```python
from build123d import *

# Parameters (mm, degrees)
F1_DEPTH       = 59.9186
F2_D           = 6.5024
F2_DEPTH       = 59.9186
F2_CSINK_D     = 7.62
F2_CSINK_ANGLE = 82
F2_TIP         = 1.9535180446
F3_R           = 3.2512
F4_DEPTH       = 50.8
F5_W           = 89.9922
F5_H           = 89.9922
F6_DEPTH       = 40.64
F7_R           = 6.35
F8_DEPTH       = 25.4
F9_R           = 36.576
F10_DEPTH      = 2.9972
F11_R          = 6.35
F12_DEPTH      = 31.75
F14_D          = 3.7973
F14_DEPTH      = 19.1008
F14_TIP        = 1.1408240143
F13_R          = 36.83
F15_DEPTH      = 1.905


with BuildPart() as f1:
    # F0 (on Front) → F1 (new body)
    with BuildSketch(Plane.XZ):
        Polygon((44.9961, 37.0295594098), (37.0295594098, 44.9961), (-37.0295594098, 44.9961), (-44.9961, 37.0295594098), (-44.9961, -37.0295594098), (-37.0295594098, -44.9961), (37.0295594098, -44.9961), (44.9961, -37.0295594098), align=None)
    extrude(amount=-F1_DEPTH)

    # F2
    with Locations(Plane.XZ):
        with Locations((-35.3552683486, 35.3552683486), (-35.3552683486, -35.3552683486), (35.3552683486, -35.3552683486), (35.3552683486, 35.3552683486)):
            CounterSinkHole(F2_D / 2, F2_CSINK_D / 2, depth=F2_DEPTH, counter_sink_angle=F2_CSINK_ANGLE)
            with Locations((0, 0, -(F2_DEPTH + F2_TIP / 2))):  # 118° drill point
                Cone(0, F2_D / 2, F2_TIP, mode=Mode.SUBTRACT)

    # F3 (on face) → F4 (cut)
    with BuildSketch(Plane(origin=(0, 59.9186, 0), x_dir=(-1, 0, 0), z_dir=(0, 1, 0))):
        with BuildLine():
            Line((-44.9961, 37.0295594098), (-44.9961, 25.4))
            ThreePointArc((-44.9961, 25.4), (-29.5424518432, 29.5424518432), (-25.4, 44.9961))
            Line((-25.4, 44.9961), (-37.0295594098, 44.9961))
            Line((-37.0295594098, 44.9961), (-44.9961, 37.0295594098))
        make_face()
        with Locations((-35.3552683486, 35.3552683486)):
            Circle(F3_R, mode=Mode.SUBTRACT)
        with BuildLine():
            ThreePointArc((44.9961, -25.4), (29.5424518432, -29.5424518432), (25.4, -44.9961))
            Line((25.4, -44.9961), (37.0295594098, -44.9961))
            Line((37.0295594098, -44.9961), (44.9961, -37.0295594098))
            Line((44.9961, -37.0295594098), (44.9961, -25.4))
        make_face()
        with Locations((35.3552683486, -35.3552683486)):
            Circle(F3_R, mode=Mode.SUBTRACT)
        with BuildLine():
            ThreePointArc((-25.4, -44.9961), (-29.5424518432, -29.5424518432), (-44.9961, -25.4))
            Line((-44.9961, -25.4), (-44.9961, -37.0295594098))
            Line((-44.9961, -37.0295594098), (-37.0295594098, -44.9961))
            Line((-37.0295594098, -44.9961), (-25.4, -44.9961))
        make_face()
        with Locations((-35.3552683486, -35.3552683486)):
            Circle(F3_R, mode=Mode.SUBTRACT)
        with BuildLine():
            Line((37.0295594098, 44.9961), (25.4, 44.9961))
            ThreePointArc((25.4, 44.9961), (29.5424518432, 29.5424518432), (44.9961, 25.4))
            Line((44.9961, 25.4), (44.9961, 37.0295594098))
            Line((44.9961, 37.0295594098), (37.0295594098, 44.9961))
        make_face()
        with Locations((35.3552683486, 35.3552683486)):
            Circle(F3_R, mode=Mode.SUBTRACT)
    extrude(amount=-F4_DEPTH, mode=Mode.SUBTRACT)

    # F5 (on face) → F6 (join)
    with BuildSketch(Plane(origin=(0, 59.9186, 0), x_dir=(-1, 0, 0), z_dir=(0, 1, 0))):
        Rectangle(F5_W, F5_H)
    extrude(amount=F6_DEPTH)

    # F7 (on face) → F8 (cut)
    with BuildSketch(Plane(origin=(0, 100.5586, 0), x_dir=(-1, 0, 0), z_dir=(0, 1, 0))):
        Circle(F7_R)
    extrude(amount=-F8_DEPTH, mode=Mode.SUBTRACT)

    # F9 (on face) → F10 (join)
    with BuildSketch(Plane.XZ):
        Circle(F9_R)
    extrude(amount=F10_DEPTH)

    # F11 (on face) → F12 (join)
    with BuildSketch(Plane.XZ.offset(2.9972)):
        Circle(F11_R)
    extrude(amount=F12_DEPTH)

    # F14
    with Locations(Plane(origin=(0, 100.5586, 0), x_dir=(-1, 0, 0), z_dir=(0, 1, 0))):
        with Locations((-34.8074727253, 34.8074727253), (-34.8074727253, -34.8074727253), (34.8074727253, -34.8074727253), (34.8074727253, 34.8074727253)):
            Hole(F14_D / 2, depth=F14_DEPTH)
            with Locations((0, 0, -(F14_DEPTH + F14_TIP / 2))):  # 118° drill point
                Cone(0, F14_D / 2, F14_TIP, mode=Mode.SUBTRACT)

    # F13 (on face) → F15 (cut)
    with BuildSketch(Plane(origin=(0, 100.5586, 0), x_dir=(-1, 0, 0), z_dir=(0, 1, 0))):
        Circle(F13_R)
    extrude(amount=-F15_DEPTH, mode=Mode.SUBTRACT)


solid = f1.part
```
CAD build for the part. Positions are in the model's coordinates, mm. A direction names the side the tool comes from. Round coordinates to 2 decimals unless told otherwise and drop trailing zeros. Order: outer loops, then holes, each group sorted by start corner. A loop starts at its lowest first (then second) coordinate and runs counter-clockwise, first axis right, second up. Notation, with made-up numbers: (56, -1) - (81, -1) arc R10 ccw to (81, 3) - close; hole circle Ø8 at (58.25, 2.5). An arc over 180 degrees is marked (long way). Answer in a Markdown table with one row per item. Add a question column.
(1) Band-saw the part on A-A on x = 0. List the corners of the cut face in (y, z).
(2) Drop flat-ended pins along their axis: pin 1 Ø4.5 at (x, z) = (-34.81, 34.81) entering from -Y; pin 2 Ø22 at (x, z) = (15, 1) entering from +Y; pin 3 Ø3.5 at (x, z) = (34.81, 34.81) entering from +Y. Give the stop position or say it passes through.
(3) Band-saw the part on C-C on y = 56. List the corners of the cut face in (x, z).
(4) Mould opens along X. For faces 6 (the face through (-21, 0, 31)), 7 (the face through (34.56, 90.87, 36.69)), 8 (the face through (44.996, 61, -1)), 9 (the face through (35.069, 80.515, -35.008)) say: +X half, -X half, draft (parallel to the pull), parting line (faces both ways), or undercut.
(5) Band-saw the part on D-D on z = 19. List the corners of the cut face in (x, y).
(6) 3-axis set-ups, long thin cutter, end or side, ignore diameter. For faces 1 (the face through (40.957, 4.495, -41.069)), 2 (the face through (1.38, 87.07, -6.2)), 3 (the face through (-29.71, 34.87, -29.38)), 4 (the face through (21, 100.559, 31)), 5 (the face through (-38.456, 4.94, 36.332)): which of +Z, -Z, +X, -X, +Y, -Y reach the whole face in a straight line?
(7) Band-saw the part on B-B on z = 0. List the corners of the cut face in (x, y), and give its area (3 significant figures).
(8) Probe L1, parallel to Z at x = 0, y = 99; L2, parallel to Z at x = 0, y = 84; L3, parallel to Y at x = 21, z = -22.5. List the from-to ranges inside material, lowest first. Write a range as [from, to].
Data:
| question | item | result |
|---|---|---|
| 1 | outline | (-34.75, -6.35) - (-3, -6.35) - (-3, -36.58) - (0, -36.58) - (0, -45) - (100.56, -45) - (100.56, -36.83) - (98.65, -36.83) - (98.65, -6.35) - (75.16, -6.35) - (75.16, 6.35) - (98.65, 6.35) - (98.65, 36.83) - (100.56, 36.83) - (100.56, 45) - (0, 45) - (0, 36.58) - (-3, 36.58) - (-3, 6.35) - (-34.75, 6.35) - close |
| 2 | pin 1 | stops at y = 59.92 |
| 2 | pin 2 | stops at y = 98.65 |
| 2 | pin 3 | stops at y = 81.37 |
| 3 | outline | (-45, -25.4) arc R16 cw to (-25.4, -45) - (25.4, -45) arc R16 cw to (45, -25.4) - (45, 25.4) arc R16 cw to (25.4, 45) - (-25.4, 45) arc R16 cw to (-45, 25.4) - close |
| 4 | face 6 | draft |
| 4 | face 7 | undercut |
| 4 | face 8 | +X half |
| 4 | face 9 | undercut |
| 5 | outline | (-45, 0) - (-31.25, 0) - (-31.25, -3) - (31.25, -3) - (31.25, 0) - (45, 0) - (45, 100.56) - (31.55, 100.56) - (31.55, 98.65) - (-31.55, 98.65) - (-31.55, 100.56) - (-45, 100.56) - close |
| 6 | face 1 | -Z, +X, -Y |
| 6 | face 2 | +Y |
| 6 | face 3 | none |
| 6 | face 4 | +Z, -Z, +X, -X, +Y |
| 6 | face 5 | -Y |
| 7 | outline | (-45, 0) - (-36.58, 0) - (-36.58, -3) - (-6.35, -3) - (-6.35, -34.75) - (6.35, -34.75) - (6.35, -3) - (36.58, -3) - (36.58, 0) - (45, 0) - (45, 100.56) - (36.83, 100.56) - (36.83, 98.65) - (6.35, 98.65) - (6.35, 75.16) - (-6.35, 75.16) - (-6.35, 98.65) - (-36.83, 98.65) - (-36.83, 100.56) - (-45, 100.56) - close |
| 7 | area | 9,230 mm^2 |
| 8 | L1 | z = [-45, -36.83], [36.83, 45] |
| 8 | L2 | z = [-45, -6.35], [6.35, 45] |
| 8 | L3 | y = [-3, 98.65] |
